Design review of the part built by this model. Coordinates are the model's own, in mm. A direction names the side the tool comes from. Coordinates: 2 decimals unless noted, no trailing zeros. Loops run counter-clockwise (first coordinate to the right, second up) from the corner with the lowest first, then second, coordinate; pieces in that order, holes last. Notation, with made-up numbers: (-32, 81) - (16, 81) arc R6 ccw to (16, 88) - close; hole circle Ø9 at (76.25, 11). An arc over 180 degrees is marked (long way). Use one line per item in the form item = value. Start each with the question number.
(1) Tool access review of faces 4 (the face through (0, 1, -2.5)), 5 (the face through (0, -2.5, -1)), 6 (the face through (0, 2.5, 1)): name each direction out of +Z, -Z, +X, -X, +Y, -Y from which nothing blocks a thin tool from reaching the whole face with its end or side.
(2) Clearance check with flat-ended pins moving along their axes: pin 1 Ø1.5 at (x, y) = (8.5, 2) entering from -Z; pin 2 Ø3 at (x, z) = (7, -1) entering from +Y; pin 3 Ø0.9 at (y, z) = (-0.5, -2.5) entering from +X. State where each tip first meets the part, or that it passes through.
(3) For L1, parallel to X at y = -2.5, z = 0.6; L2, parallel to X at y = 1.65, z = 1.95; L3, parallel to Z at x = 1.75, y = 1.4, list the stretches that pass through material, from the lowest coordinate up.
(4) Add section C-C (x = 2). State the section outline as (y, z) points, plus the area to 3 significant figures.
(5) The part is to be moulded in two halves that separate along Y. For faces 1 (the face through (6.034, 1.468, -1.915)), 2 (the face through (0, 2.52, -0.9)), 3 (the face through (0, -1, 2.5)), say which applies: pulls with the +Y half, pulls with the -Y half, needs draft (parallel to the pull), parting line crosses it, or undercut.
```python
from build123d import *

# Parameters (mm, degrees)
RIBCUT_START     = -0.428625
RIBCUT_DEPTH     = 0.428625
RIBCUTSPAT_COUNT = 8
RIBCUTSPAT_ANGLE = 315


with BuildPart() as part:
    # BodySke → BaseBody (revolve)
    with BuildSketch(Plane.XY, mode=Mode.PRIVATE) as basebody_sk:
        with BuildLine():
            Line((-0.428625, 2.74066), (-0.428625, 0))
            Line((-0.428625, 0), (12.271375, 0))
            Line((12.271375, 0), (12.271375, 1.94056))
            Line((12.271375, 1.94056), (11.798935, 2.413))
            Line((11.798935, 2.413), (0.428625, 2.413))
            Line((0.428625, 2.413), (0.428625, 2.701493258))
            Line((0.428625, 2.701493258), (0, 2.8575))
            Line((0, 2.8575), (-0.311785, 2.8575))
            ThreePointArc((-0.311785, 2.8575), (-0.392607305, 2.824022305), (-0.426085, 2.7432))
            Line((-0.426085, 2.7432), (-0.426085, 2.74066))
            Line((-0.426085, 2.74066), (-0.428625, 2.74066))
        make_face()
    revolve(basebody_sk.sketch.rotate(Axis((0, 0, 0), (1, 0, 0)), 90), axis=Axis((0, 0, 0), (1, 0, 0)))

    # RibCutSke → RibCut (cut)
    with BuildSketch(Plane(origin=(0.428625, 1.794401132, -0.090952894), x_dir=(0, 0, -1), z_dir=(1, 0, 0)).offset(RIBCUT_START)):
        with BuildLine():
            Line((0.224006808, 0.70999648), (0.224006808, 1.045688063))
            ThreePointArc((0.224006808, 1.045688063), (1.002565014, 0.845584632), (1.694583294, 0.436555338))
            Line((1.694583294, 0.436555338), (1.4572135, 0.199185543))
            ThreePointArc((1.4572135, 0.199185543), (0.874987925, 0.537586293), (0.224006808, 0.70999648))
        make_face()
    ribcut = extrude(amount=RIBCUT_DEPTH, mode=Mode.SUBTRACT)

    # RibCutsPat: RibCut ×8 about axis
    ribcutspat_axis = Axis((0, 0, 0), (1, 0, 0))
    for i in range(1, RIBCUTSPAT_COUNT):
        add(ribcut.rotate(ribcutspat_axis, i * RIBCUTSPAT_ANGLE / (RIBCUTSPAT_COUNT - 1)), mode=Mode.SUBTRACT)


solid = part.part
```
Computed values:
q1.face_4 = -Z, +X
q1.face_5 = +X, -Y
q1.face_6 = +X, +Y
q2.pin_1 = -2.06
q2.pin_2 = 2.41
q2.pin_3 = 12.11
q3.L1 = -0.43 to 0
q3.L2 = -0.43 to 0.43
q3.L3 = -1.97 to 1.97
q4.outline = circle Ø4.83 at (0, 0)
q4.area = 18.3 mm^2
q5.face_1 = parting line crosses it
q5.face_2 = needs draft
q5.face_3 = undercut
